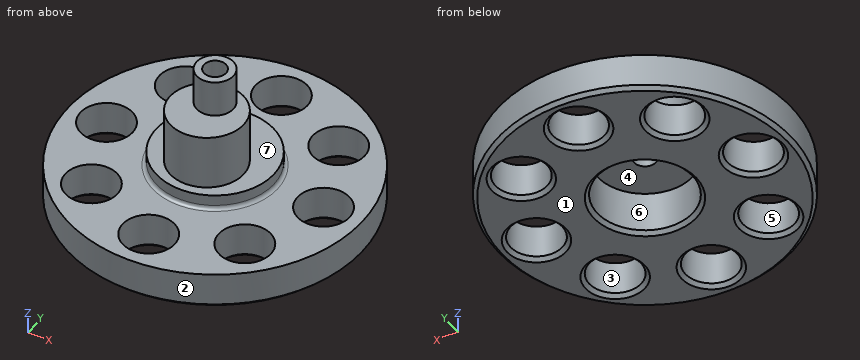
from build123d import *

# Parameters (mm, degrees)
SKETCH1_R           = 20
SKETCH1_R_2         = 3.54
BOSS_EXTRUDE1_DEPTH = 5
SKETCH2_R           = 8
BOSS_EXTRUDE2_DEPTH = 2
SKETCH3_R           = 6.5
CUT_EXTRUDE1_DEPTH  = 6
SKETCH4_R           = 5
BOSS_EXTRUDE3_DEPTH = 7.5
SKETCH5_R           = 2.5
BOSS_EXTRUDE4_DEPTH = 5
FILLET1_R           = 0.5
CHAMFER1_SIZE       = 0.5
SKETCH7_R           = 1.5
CUT_EXTRUDE2_DEPTH  = 15


with BuildPart() as part:
    # Sketch1 → Boss-Extrude1 (new body)
    with BuildSketch(Plane.XY):
        Circle(SKETCH1_R)
        with Locations((-14.783956386, 0)):
            Circle(SKETCH1_R_2, mode=Mode.SUBTRACT)
        with Locations((-10.453835814, -10.453835814)):
            Circle(SKETCH1_R_2, mode=Mode.SUBTRACT)
        with Locations((0, -14.783956386)):
            Circle(SKETCH1_R_2, mode=Mode.SUBTRACT)
        with Locations((10.453835814, -10.453835814)):
            Circle(SKETCH1_R_2, mode=Mode.SUBTRACT)
        with Locations((14.783956386, 0)):
            Circle(SKETCH1_R_2, mode=Mode.SUBTRACT)
        with Locations((10.453835814, 10.453835814)):
            Circle(SKETCH1_R_2, mode=Mode.SUBTRACT)
        with Locations((0, 14.783956386)):
            Circle(SKETCH1_R_2, mode=Mode.SUBTRACT)
        with Locations((-10.453835814, 10.453835814)):
            Circle(SKETCH1_R_2, mode=Mode.SUBTRACT)
    extrude(amount=BOSS_EXTRUDE1_DEPTH)

    # Sketch2 → Boss-Extrude2 (add)
    with BuildSketch(Plane.XY.offset(5)):
        Circle(SKETCH2_R)
    extrude(amount=BOSS_EXTRUDE2_DEPTH)

    # Sketch3 → Cut-Extrude1 (cut)
    with BuildSketch(Plane(origin=(0, 0, 0), x_dir=(-1, 0, 0), z_dir=(0, 0, -1))):
        Circle(SKETCH3_R)
    extrude(amount=-CUT_EXTRUDE1_DEPTH, mode=Mode.SUBTRACT)

    # Sketch4 → Boss-Extrude3 (add)
    with BuildSketch(Plane.XY.offset(7)):
        with Locations((0, -1.812)):
            Circle(SKETCH4_R)
    extrude(amount=BOSS_EXTRUDE3_DEPTH)

    # Sketch5 → Boss-Extrude4 (add)
    with BuildSketch(Plane.XY.offset(14.5)):
        Circle(SKETCH5_R)
    extrude(amount=BOSS_EXTRUDE4_DEPTH)

    # Fillet1
    fillet1_edges = [part.edges().sort_by_distance(p)[0] for p in [
        (-8, 0, 5),
    ]]
    fillet(fillet1_edges, radius=FILLET1_R)

    # Chamfer1
    chamfer1_edges = [part.edges().sort_by_distance(p)[0] for p in [
        (-3.54, -14.783956386, 0),
        (6.913835814, -10.453835814, 0),
        (-20, 0, 0),
        (11.243956386, 0, 0),
        (6.913835814, 10.453835814, 0),
        (-3.54, 14.783956386, 0),
        (-13.993835814, 10.453835814, 0),
        (6.5, 0, 0),
        (-18.323956386, 0, 0),
        (-13.993835814, -10.453835814, 0),
    ]]
    chamfer(chamfer1_edges, length=CHAMFER1_SIZE)

    # Sketch7 → Cut-Extrude2 (cut)
    with BuildSketch(Plane.XY.offset(19.5)):
        Circle(SKETCH7_R)
    extrude(amount=-CUT_EXTRUDE2_DEPTH, mode=Mode.SUBTRACT)


solid = part.part
Read the model definition and answer for the solid it produces. Units are mm, in the model's axes. Face numbers are marked on the shaded views. A direction names the side the tool comes from. Give positions to 0.01 mm unless a question says otherwise; leave off trailing zeros. Write each loop counter-clockwise with the first axis right and the second up, starting at its lowest first coordinate (ties: lowest second). Pieces come first, ordered by that corner, then holes. Notation, with made-up numbers: (60.5, 88.5) - (85.5, 88.5) arc R9 ccw to (85.5, 103.5) - close; hole circle Ø9 at (55.25, 67.25). An arc over 180 degrees is marked (long way). Return JSON: item names as keys, results as strings.
Q1. A cutting plane is placed at A-A, the plane z = 2. Count the separate pieces of the cut face and the enclosed holes in it, and give its area (3 significant figures).
Reply:
{"separate pieces": "1", "enclosed holes": "9", "area": "809 mm²"}
Q2. Consider line 1 along Y through (x, z) = (0, 2.1); line 2 along Z through (x, y) = (7, 17); line 3 along X through (y, z) = (-5, 1). Determine where each line is inside the solid, lowest interval first. Write a range as [from, to].
Reply:
{"line 1": "[-20, -18.32], [-11.24, -6.5], [6.5, 11.24], [18.32, 20]", "line 2": "[0, 5]", "line 3": "[-19.36, -4.15], [4.15, 19.36]"}
Q3. A cutting plane is placed at C-C, the plane z = 18.25. Determine the outline of the cut face in (x, y).
Reply:
{"outline": "circle Ø5 at (0, 0); hole circle Ø3 at (0, 0)"}
Q4. For a pull along Y with two mould halves and no side action, classify the marked faces 1, 2, 3 and 4 as released by +Y, released by -Y, zero draft, split by the parting line, or undercut.
Reply:
{"face 1": "zero draft", "face 2": "split by the parting line", "face 3": "undercut", "face 4": "undercut"}
Q5. Given P1, Ø11.5, axis at x = 14.78, y = 0, coming from the +Z side; P2, Ø8, axis at x = -9, z = 8, coming from the +Y side; P3, Ø8, axis at x = -14.78, y = 0, coming from the -Z side, each flat-ended and moving along its own axis, determine where each tip first touches the part or whether it passes through.
Reply:
{"P1": "z = 5", "P2": "y = 18.96", "P3": "z = 0.04"}
Q6. For the marked faces 5, 6 and 7, determine the directions among +Z, -Z, +X, -X, +Y, -Y from which every point of the face is accessible in a straight line to the end or side of a thin tool.
Reply:
{"face 5": "+Z, -Z", "face 6": "-Z", "face 7": "+Z"}
